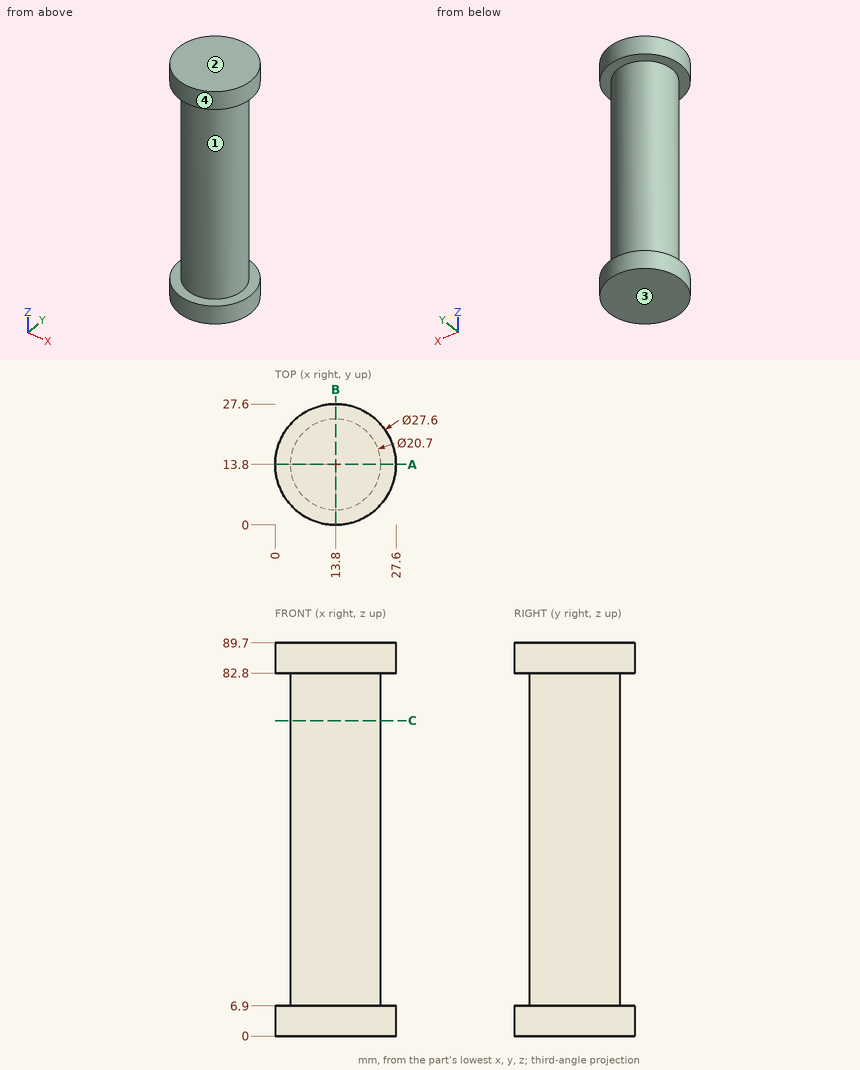
Can you work these out from the drawing? Everything is in mm from the part's minimum corner. Round coordinates to 2 decimals unless told otherwise and drop trailing zeros. Write each loop counter-clockwise with the first axis right and the second up, starting at its lowest first coordinate (ties: lowest second). Pieces come first, ordered by that corner, then holes. Notation, with made-up numbers: (79, -36.5) - (87, -36.5) arc R19 ccw to (87, -3.5) - close; hole circle Ø7 at (-12.75, 75.25). An arc over 180 degrees is marked (long way). Use a Markdown table: item, result.
Q1. Please list where these lines run through material, in increasing order: L1, parallel to Z at x = 24.5, y = 9.5; L2, parallel to X at y = 20.5, z = 66; L3, parallel to Y at x = 11, z = 34.
Output values:
| item | result |
|---|---|
| L1 | 0 to 6.9, 82.8 to 89.7 |
| L2 | 5.91 to 21.69 |
| L3 | 3.84 to 23.76 |
Q2. Thinking about a two-plate mould opening in Z: for the marked faces 1, 2, 3 and 4, which applies, released by +Z, released by -Z, zero draft, split by the parting line, or undercut?
Output values:
| item | result |
|---|---|
| face 1 | undercut |
| face 2 | released by +Z |
| face 3 | released by -Z |
| face 4 | zero draft |
Q3. For pin 1 (10 mm diameter, centred on y = 22.5, z = 21, fed in from -X); pin 2 (12 mm diameter, centred on x = 5, z = 60.5, fed in from +Y); pin 3 (8 mm diameter, centred on y = 14.5, z = 76, fed in from -X), each with a flat end and sliding along its axis, tell me the tip position at first contact or that it passes through.
Output values:
| item | result |
|---|---|
| pin 1 | x = 4.13 |
| pin 2 | y = 23.76 |
| pin 3 | x = 3.45 |
Q4. I want a section at A-A (y = 13.8). List the corners of the cut face in (x, z) for me, plus the area to 3 significant figures.
Output values:
| item | result |
|---|---|
| outline | (0, 0) - (27.6, 0) - (27.6, 6.9) - (24.15, 6.9) - (24.15, 82.8) - (27.6, 82.8) - (27.6, 89.7) - (0, 89.7) - (0, 82.8) - (3.45, 82.8) - (3.45, 6.9) - (0, 6.9) - close |
| area | 1,950 mm2 |
Q5. I want a section at C-C (z = 72). List the corners of the cut face in (x, y) for me, plus the area to 3 significant figures.
Output values:
| item | result |
|---|---|
| outline | circle Ø20.7 at (13.8, 13.8) |
| area | 337 mm2 |
